Can you work these out from the drawing? Everything is in mm from the part's minimum corner. A direction names the side the tool comes from. Round coordinates to 2 decimals unless told otherwise and drop trailing zeros. Order: outer loops, then holes, each group sorted by start corner. A loop starts at its lowest first (then second) coordinate and runs counter-clockwise, first axis right, second up. Notation, with made-up numbers: (-15, 7.25) - (-8, 7.25) arc R13 cw to (-8, 24.25) - close; hole circle Ø5 at (47, 87). An arc over 180 degrees is marked (long way). Answer as a JSON object with one key per item and string values.
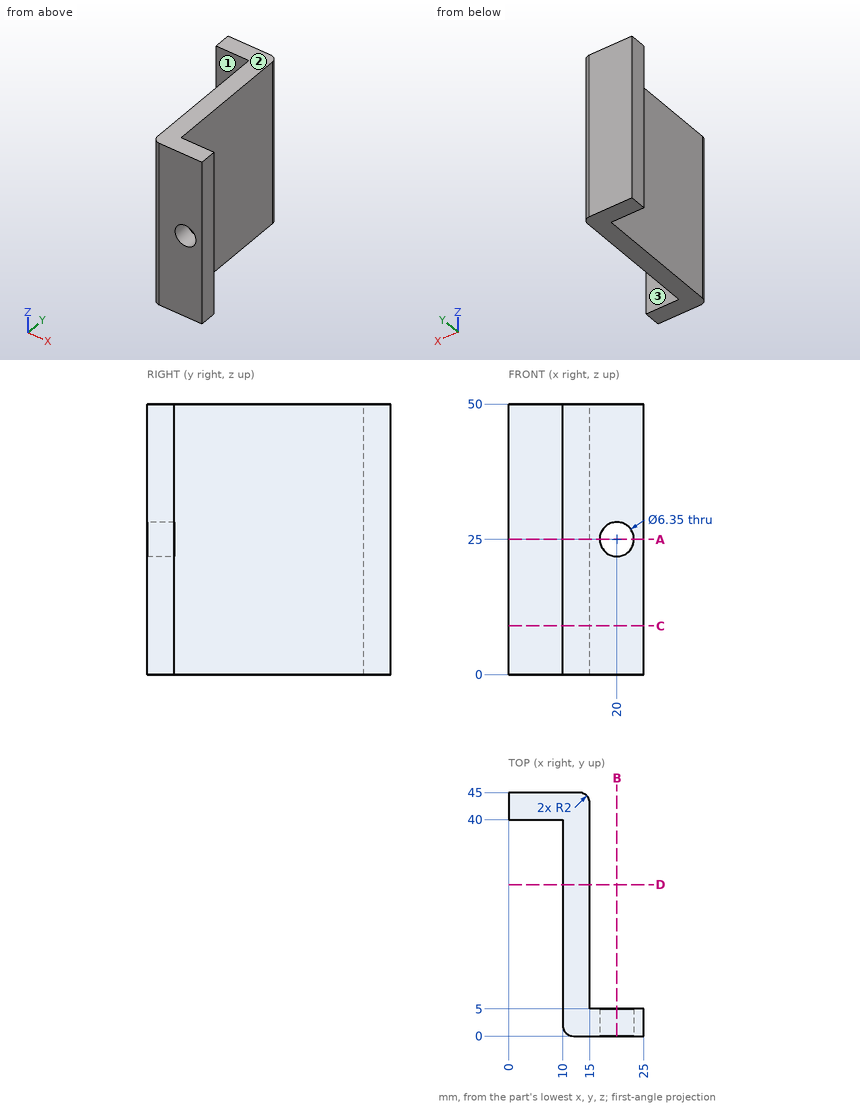
1. For the marked faces 1, 2 and 3, which set-ups out of +Z, -Z, +X, -X, +Y, -Y let a thin tool reach every point of the face, with its end or its side?
Responses:
{"face 1": "+Z, -Z, -X, -Y", "face 2": "+Z, +X, -X, +Y, -Y", "face 3": "+Z, -Z, +X, +Y"}
2. For P1, Ø11, axis at x = 21.5, z = 17, coming from the +Y side; P2, Ø4, axis at x = 12, y = 11, coming from the -Z side; P3, Ø5, axis at x = 6.5, z = 14, coming from the -Y side; P4, Ø2, axis at y = 9.5, z = 8, coming from the +X side, each with a flat end and sliding along its axis, tell me the tip position at first contact or that it passes through.
Responses:
{"P1": "y = 5", "P2": "z = 0", "P3": "y = 40", "P4": "x = 15"}
3. If I drill on L1, parallel to X at y = 2.25, z = 25 (3 decimals); L2, parallel to Y at x = 23.75, z = 23; L3, parallel to X at y = 1, z = 25 (3 decimals), over which ranges is the centre line in solid material (lowest first)? Write a range as [from, to].
Responses:
{"L1": "[10, 16.825], [23.175, 25]", "L2": "[0, 5]", "L3": "[10.268, 16.825], [23.175, 25]"}
4. Imagine slicing it at A-A (z = 25). List the corners of the cut face in (x, y) for me (3 decimals).
Responses:
{"outline": "(0, 40) - (10, 40) - (10, 2) arc R2 ccw to (12, 0) - (16.825, 0) - (16.825, 5) - (15, 5) - (15, 43) arc R2 ccw to (13, 45) - (0, 45) - close; (23.175, 0) - (25, 0) - (25, 5) - (23.175, 5) - close"}
5. Imagine slicing it at B-B (x = 20). List the corners of the cut face in (y, z) for me (3 decimals), plus the area to 3 significant figures.
Responses:
{"outline": "(0, 0) - (5, 0) - (5, 21.825) - (0, 21.825) - close; (0, 28.175) - (5, 28.175) - (5, 50) - (0, 50) - close", "area": "218 mm2"}
6. Imagine slicing it at D-D (y = 28). List the corners of the cut face in (x, z) for me, plus the area to 3 significant figures.
Responses:
{"outline": "(10, 0) - (15, 0) - (15, 50) - (10, 50) - close", "area": "250 mm2"}
7. Imagine slicing it at C-C (z = 9). List the corners of the cut face in (x, y) for me.
Responses:
{"outline": "(0, 40) - (10, 40) - (10, 2) arc R2 ccw to (12, 0) - (25, 0) - (25, 5) - (15, 5) - (15, 43) arc R2 ccw to (13, 45) - (0, 45) - close"}
